from build123d import *

# Parameters (mm, degrees)
SKETCH1_R           = 3.5941
BOSS_EXTRUDE1_DEPTH = 3.8862
SKETCH2_R           = 2.7051
CUT_EXTRUDE1_DEPTH  = 3.8862
FILLET1_R           = 0.4445
FILLET2_R           = 0.4445


with BuildPart() as part:
    # Sketch1 → Boss-Extrude1 (new body)
    with BuildSketch(Plane(origin=(0, 0, 0), x_dir=(1, 0, 0), z_dir=(0, 1, 0))):
        with Locations(Location((0, 0, 0), (0, 0, 90))):
            Circle(SKETCH1_R)
    extrude(amount=BOSS_EXTRUDE1_DEPTH)

    # Sketch2 → Cut-Extrude1 (cut)
    with BuildSketch(Plane(origin=(0, 3.8862, 0), x_dir=(1, 0, 0), z_dir=(0, 1, 0))):
        with Locations(Location((0, 0, 0), (0, 0, 270))):
            Circle(SKETCH2_R)
    extrude(amount=-CUT_EXTRUDE1_DEPTH, mode=Mode.SUBTRACT)

    # Fillet1
    fillet1_edges = [part.edges().sort_by_distance(p)[0] for p in [
        (0, 3.8862, 3.5941),
        (0, 3.8862, -2.7051),
    ]]
    fillet(fillet1_edges, radius=FILLET1_R - 0.0001)  # a hair under: the kernel refuses the full size

    # Fillet2
    fillet2_edges = [part.edges().sort_by_distance(p)[0] for p in [
        (0, 0, 3.5941),
        (0, 0, -2.7051),
    ]]
    fillet(fillet2_edges, radius=FILLET2_R - 0.0001)  # a hair under: the kernel refuses the full size


solid = part.part
The model under review builds one solid part; all positions refer to its coordinate system, in mm. Round coordinates to 2 decimals unless told otherwise and drop trailing zeros. Order: outer loops, then holes, each group sorted by start corner. A loop starts at its lowest first (then second) coordinate and runs counter-clockwise, first axis right, second up. Notation, with made-up numbers: (67, -39) -> (113, -39) arc R27 cw to (113, -19) -> close; hole circle Ø11 at (19, 49). An arc over 180 degrees is marked (long way). Write item = value, one per line. Start each with the question number.
Item 1: Clearance check with a flat-ended pin moving along its axis: pin 1 Ø1 at (y, z) = (3, 2) entering from +X. State where the tip first meets the part, or that it passes through.
Item 2: Consider section C-C on y = 3.25. Write out the cut boundary in (x, z), plus the area to 3 significant figures.
Item 3: For line 1 along X through (y, z) = (2.4, 0); line 2 along Z through (x, y) = (-2.25, 3.2), list the stretches that pass through material, from the lowest coordinate up.
Item 4: Mouldability with a two-part tool opening along X and no side actions: class faces 1 (the face through (0.81, 1.96, 2.58)), 2 (the face through (-3.564, 1.922, 0.468)) as released by +X, released by -X, zero draft, split by the parting line, or undercut.
Conclusion:
q1.pin_1 = 3.27
q2.outline = circle Ø7.19 at (0, 0); hole circle Ø5.41 at (0, 0)
q2.area = 17.6 mm2
q3.line_1 = -3.59 to -2.71, 2.71 to 3.59
q3.line_2 = -2.8 to -1.5, 1.5 to 2.8
q4.face_1 = undercut
q4.face_2 = split by the parting line
